from build123d import *

# Parameters (mm, degrees)
SKETCH_1_W          = 250
SKETCH_1_H          = 100
EXTRUDE_1_DEPTH     = 370
CUT_EXTRUDE_1_DEPTH = 370
CUT_EXTRUDE_3_DEPTH = 458.602447546


with BuildPart() as part:
    # 草圖1 → 填料-伸長1 (new body)
    with BuildSketch(Plane.XY):
        Rectangle(SKETCH_1_W, SKETCH_1_H)
    extrude(amount=EXTRUDE_1_DEPTH)

    # 草圖2 → 除料-伸長1 (cut)
    with BuildSketch(Plane.XY.offset(370)):
        Polygon((-125, 50), (-100, -50), (-125, -50), align=None)
        Polygon((125, 50), (125, -50), (100, -50), align=None)
    extrude(amount=-CUT_EXTRUDE_1_DEPTH, mode=Mode.SUBTRACT)

    # 草圖7 → 除料-伸長3 (cut, through all)
    with BuildSketch(Plane(origin=(-125, 50, 370), x_dir=(0, 0, 1), z_dir=(-1, 0, 0))):
        Polygon((0, 0), (-15, -100), (0, -100), align=None)
        Polygon((-370, 0), (-265, -100), (-370, -100), align=None)
    extrude(amount=-CUT_EXTRUDE_3_DEPTH, mode=Mode.SUBTRACT)


solid = part.part
Can you work these out from the model? Positions are in its coordinate system, mm. Round coordinates to 2 decimals unless told otherwise and drop trailing zeros. Write each loop counter-clockwise with the first axis right and the second up, starting at its lowest first coordinate (ties: lowest second). Pieces come first, ordered by that corner, then holes. Notation, with made-up numbers: (13.5, -22) -> (38.5, -22) arc R8 cw to (38.5, -13) -> close; hole circle Ø8 at (24, 58.25). An arc over 180 degrees is marked (long way). One line per question, with ' | ' between items. Start each with the question number.
1) Suppose I cut it at A-A on y = -13. Write out the boundary of the cut face in (x, z), then the cut area to 3 significant figures.
2) I need wall thicknesses on line 1 (Z direction, x = 109, y = 31); line 2 (X direction, y = 16.5, z = 129) (3 decimals); line 3 (Z direction, x = 109, y = 46). Which ranges of each line are inside material? Lowest first, please. Write a range as [from, to].
3) I'm going to push flat-ended pins straight in: P1, Ø3, axis at x = -79.5, y = 16.5, coming from the +Z side; P2, Ø1.5, axis at y = -20, z = 148.5, coming from the +X side; P3, Ø8, axis at x = -13, y = 36, coming from the -Z side. Where does each tip first touch, or does it pass through?
4) Suppose I cut it at B-B on z = 73.5. Write out the boundary of the cut face in (x, y), then the cut area to 3 significant figures.
Return value:
1) outline: (-109.25, 66.15) -> (109.25, 66.15) -> (109.25, 360.55) -> (-109.25, 360.55) -> close | area: 64,300 mm2
2) line 1: z = [19.95, 367.15] | line 2: x = [-116.625, 116.625] | line 3: z = [4.2, 369.4]
3) P1: stops at z = 365.2 | P2: stops at x = 107.69 | P3: stops at z = 10.5
4) outline: (-125, 50) -> (-107.5, -20) -> (107.5, -20) -> (125, 50) -> close | area: 16,300 mm2
